Geometry check sheet. Reference: the model listing, model coordinates, mm. Coordinates: 2 decimals unless noted, no trailing zeros. Write each loop counter-clockwise with the first axis right and the second up, starting at its lowest first coordinate (ties: lowest second). Pieces come first, ordered by that corner, then holes. Notation, with made-up numbers: (39, -34) -> (95, -34) arc R14 ccw to (95, -23) -> close; hole circle Ø11 at (28, 46.25). An arc over 180 degrees is marked (long way). Answer in a Markdown table with one row per item. Add a question column.
Q1. Section check A-A, the plane x = 35. Record the boundary of the cut face in (y, z) (3 decimals).
Q2. Section check C-C, the plane x = 0. Record the boundary of the cut face in (y, z) (3 decimals).
Q3. Thickness scan on line 1 (X direction, y = 0.8, z = 10); line 2 (X direction, y = 2.45, z = 0); line 3 (Z direction, x = 85, y = 1.75). Record the ranges inside material, lowest first.
Q4. Section check B-B, the plane y = 1.2. Count the separate pieces of the cut face and the enclosed holes in it, and give its area (3 significant figures).
```python
from build123d import *

# Parameters (mm, degrees)
SKETCH1_W           = 150
SKETCH1_H           = 30
BOSS_EXTRUDE1_DEPTH = 3.175
FILLET1_R           = 5
SKETCH2_R           = 2.5
CUT_EXTRUDE1_DEPTH  = 136.867879298
SKETCH3_R           = 1.5
CUT_EXTRUDE3_DEPTH  = 136.867879298
SKETCH4_R           = 1.5
CUT_EXTRUDE4_DEPTH  = 10


with BuildPart() as part:
    # Sketch1 → Boss-Extrude1 (new body)
    with BuildSketch(Plane(origin=(0, 0, 0), x_dir=(1, 0, 0), z_dir=(0, 1, 0))):
        with Locations((60, 0)):
            Rectangle(SKETCH1_W, SKETCH1_H)
    extrude(amount=BOSS_EXTRUDE1_DEPTH)

    # Fillet1
    fillet1_edges = [part.edges().sort_by_distance(p)[0] for p in [
        (-15, 1.5875, -15),
        (135, 1.5875, -15),
        (135, 1.5875, 15),
        (-15, 1.5875, 15),
    ]]
    fillet(fillet1_edges, radius=FILLET1_R)

    # Sketch2 → Cut-Extrude1 (cut, through all)
    with BuildSketch(Plane(origin=(0, 3.175, 0), x_dir=(1, 0, 0), z_dir=(0, 1, 0))):
        with Locations(Location((0, 0, 0), (0, 0, 270))):
            Circle(SKETCH2_R)
    extrude(amount=-CUT_EXTRUDE1_DEPTH, mode=Mode.SUBTRACT)

    # Sketch3 → Cut-Extrude3 (cut, through all)
    with BuildSketch(Plane(origin=(0, 3.175, 0), x_dir=(1, 0, 0), z_dir=(0, 1, 0))):
        with Locations(Location((7.5, 0, 0), (0, 0, 270))):
            Circle(SKETCH3_R)
        with Locations(Location((0, -7.5, 0), (0, 0, 270))):
            Circle(SKETCH3_R)
        with Locations(Location((-7.5, 0, 0), (0, 0, 270))):
            Circle(SKETCH3_R)
        with Locations(Location((0, 7.5, 0), (0, 0, 270))):
            Circle(SKETCH3_R)
    extrude(amount=-CUT_EXTRUDE3_DEPTH, mode=Mode.SUBTRACT)

    # Sketch4 → Cut-Extrude4 (cut)
    with BuildSketch(Plane(origin=(0, 3.175, 0), x_dir=(1, 0, 0), z_dir=(0, 1, 0))):
        with Locations(Location((35, -10, 0), (0, 0, 270))):
            Circle(SKETCH4_R)
        with Locations(Location((85, -10, 0), (0, 0, 270))):
            Circle(SKETCH4_R)
        with Locations(Location((85, 10, 0), (0, 0, 270))):
            Circle(SKETCH4_R)
        with Locations(Location((35, 10, 0), (0, 0, 270))):
            Circle(SKETCH4_R)
    extrude(amount=-CUT_EXTRUDE4_DEPTH, mode=Mode.SUBTRACT)


solid = part.part
```
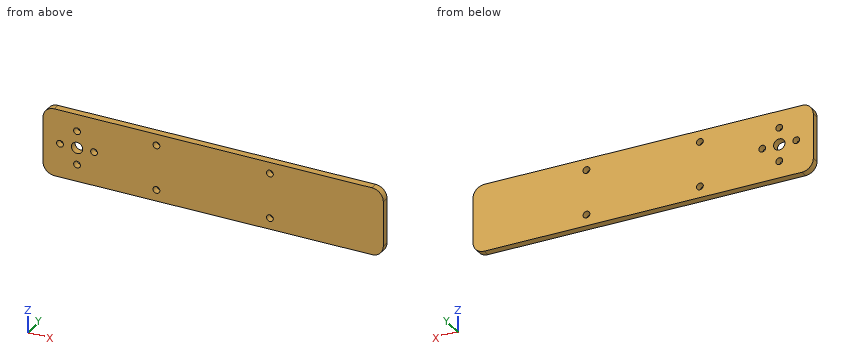
Calculated:
| question | item | result |
|---|---|---|
| 1 | outline | (0, -15) -> (3.175, -15) -> (3.175, -11.5) -> (0, -11.5) -> close; (0, -8.5) -> (3.175, -8.5) -> (3.175, 8.5) -> (0, 8.5) -> close; (0, 11.5) -> (3.175, 11.5) -> (3.175, 15) -> (0, 15) -> close |
| 2 | outline | (0, -15) -> (3.175, -15) -> (3.175, -9) -> (0, -9) -> close; (0, -6) -> (3.175, -6) -> (3.175, -2.5) -> (0, -2.5) -> close; (0, 2.5) -> (3.175, 2.5) -> (3.175, 6) -> (0, 6) -> close; (0, 9) -> (3.175, 9) -> (3.175, 15) -> (0, 15) -> close |
| 3 | line 1 | x = -15 to 33.5, 36.5 to 83.5, 86.5 to 135 |
| 3 | line 2 | x = -15 to -9, -6 to -2.5, 2.5 to 6, 9 to 135 |
| 3 | line 3 | z = -15 to -11.5, -8.5 to 8.5, 11.5 to 15 |
| 4 | separate pieces | 1 |
| 4 | enclosed holes | 9 |
| 4 | area | 4,400 mm² |
